```python
from build123d import *

# Parameters (mm, degrees)
SKETCH1_R             = 8
SKETCH1_R_2           = 4
BOSS_EXTRUDE1_DEPTH   = 9
BOSS_EXTRUDE1_2_DEPTH = 9
SKETCH2_R             = 4
BOSS_EXTRUDE3_DEPTH   = 9
FILLET1_R             = 1
SKETCH3_W             = 9
SKETCH3_H             = 9
SKETCH3_H_2           = 7
CUT_EXTRUDE1_DEPTH    = 214.789616212


with BuildPart() as part:
    # Sketch1 → Boss-Extrude1 (new body)
    with BuildSketch(Plane.XY):
        with Locations((-125, 0)):
            Circle(SKETCH1_R)
        with Locations((-125, 0)):
            Circle(SKETCH1_R_2, mode=Mode.SUBTRACT)
    extrude(amount=BOSS_EXTRUDE1_DEPTH)



with BuildPart() as body_2:
    # Sketch1 → Boss-Extrude1 2 (new body)
    with BuildSketch(Plane.XY):
        with Locations((125, 0)):
            Circle(SKETCH1_R)
        with Locations((125, 0)):
            Circle(SKETCH1_R_2, mode=Mode.SUBTRACT)
    extrude(amount=BOSS_EXTRUDE1_2_DEPTH)


with BuildPart() as part_1:
    add(part.part)

    add(body_2.part)  # Boss-Extrude3 merges body 2
    # Sketch2 → Boss-Extrude3 (add)
    with BuildSketch(Plane.XY):
        with BuildLine():
            Line((-175, -75), (125, -75))
            ThreePointArc((125, -75), (130.131670325, -43.377223009), (145.000000492, -14.999999344))
            ThreePointArc((145.000000492, -14.999999344), (143.981414944, 16.269784471), (113.235294528, 22.058823748))
            ThreePointArc((113.235294528, 22.058823748), (25.000000075, 0), (-63.235294395, 22.058823677))
            ThreePointArc((-63.235294395, 22.058823677), (-75.420498385, 24.996463372), (-87.499999896, 21.650635154))
            ThreePointArc((-87.499999896, 21.650635154), (-99.999999954, 18.301270189), (-112.500000024, 21.650635108))
            ThreePointArc((-112.500000024, 21.650635108), (-124.99999995, 25), (-137.49999989, 21.650635158))
            ThreePointArc((-137.49999989, 21.650635158), (-149.999999954, 18.301270189), (-162.50000003, 21.650635112))
            ThreePointArc((-162.50000003, 21.650635112), (-193.705072901, 16.586749162), (-195.000000551, -14.999999265))
            ThreePointArc((-195.000000551, -14.999999265), (-180.13167034, -43.377222962), (-175, -75))
        make_face()
        with Locations((125, 0)):
            Circle(SKETCH2_R, mode=Mode.SUBTRACT)
        with Locations((-175, 0)):
            Circle(SKETCH2_R, mode=Mode.SUBTRACT)
        with Locations((-125, 0)):
            Circle(SKETCH2_R, mode=Mode.SUBTRACT)
        with Locations((-75, 0)):
            Circle(SKETCH2_R, mode=Mode.SUBTRACT)
    extrude(amount=BOSS_EXTRUDE3_DEPTH)

    # Fillet1
    fillet1_edges = [part_1.edges().sort_by_distance(p)[0] for p in [
        (-175, -75, 4.5),
        (125, -75, 4.5),
    ]]
    fillet(fillet1_edges, radius=FILLET1_R)

    # Sketch3 → Cut-Extrude1 (cut, through all)
    with BuildSketch(Plane.XY):
        with Locations((-160.208548161, -70.5)):
            Rectangle(SKETCH3_W, SKETCH3_H)
        with Locations((-25.351798772, -70.5)):
            Rectangle(SKETCH3_W, SKETCH3_H)
        with Locations((109.504950616, -70.5)):
            Rectangle(SKETCH3_W, SKETCH3_H)
        with Locations((-160.208548161, -53.5)):
            Rectangle(SKETCH3_W, SKETCH3_H_2)
        with Locations((-25.351798772, -53.5)):
            Rectangle(SKETCH3_W, SKETCH3_H_2)
        with Locations((109.504950616, -53.5)):
            Rectangle(SKETCH3_W, SKETCH3_H_2)
    extrude(amount=CUT_EXTRUDE1_DEPTH, mode=Mode.SUBTRACT)


solid = part_1.part
```
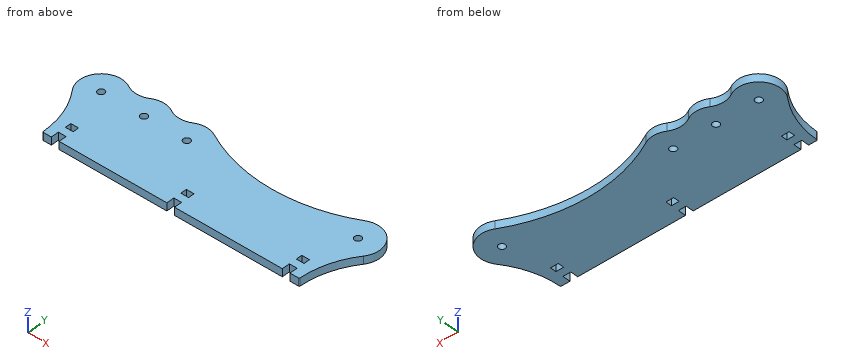
Check sheet for the modelled part. Datum: model origin and axes. Units: mm. Round coordinates to 2 decimals unless told otherwise and drop trailing zeros. Loops run counter-clockwise (first coordinate to the right, second up) from the corner with the lowest first, then second, coordinate; pieces in that order, holes last. Notation, with made-up numbers: (-23.75, 36.5) - (34.25, 36.5) arc R20 cw to (34.25, 62.5) - close; hole circle Ø10 at (-14.5, 59.5). An arc over 180 degrees is marked (long way). Answer as a JSON object with one key per item and string values. Group by question number.
Q1. Gauge pin test, flat ends, axial feed: P1, Ø4.5, axis at x = -23.5, z = 6.5, coming from the -Y side; P2, Ø2.5, axis at y = -70, z = 4, coming from the +X side; P3, Ø9, axis at x = -75, y = 0, coming from the -Z side; P4, Ø2, axis at y = -52.5, z = 6.5, coming from the +X side. Record the tip position at first contact, or that the pin passes through.
Q2. Sectioned sample at D-D, the plane y = -19. Enter the section's corners in (x, z), plus the area to 3 significant figures.
Q3. Sectioned sample at B-B, the plane x = -75. Enter the section's corners in (y, z).
Q4. Sectioned sample at A-A, the plane y = 13. Enter the section's corners in (x, z), plus the area to 3 significant figures.
Q5. Sectioned sample at C-C, the plane z = 3. Count the separate pieces of the cut face and the enclosed holes in it, plus the area to 3 significant figures.
Q6. Scan lines: line 1 along Y through (x, z) = (-125, 5); line 2 along X through (y, z) = (17.5, 6.75); line 3 along Y through (x, z) = (-151.5, 2). Record each from-to range of solid material in increasing order. Write a range as [from, to].
Solution:
{
 "1": {"P1": "stops at y = -66", "P2": "stops at x = 125.2", "P3": "stops at z = 0", "P4": "stops at x = 127.8"},
 "2": {"outline": "(-192.15, 0) - (142.15, 0) - (142.15, 9) - (-192.15, 9) - close", "area": "3,010 mm²"},
 "3": {"outline": "(-75, 0) - (-4, 0) - (-4, 9) - (-75, 9) - close; (4, 0) - (25, 0) - (25, 9) - (4, 9) - close"},
 "4": {"outline": "(-196.35, 0) - (-43.6, 0) - (-43.6, 9) - (-196.35, 9) - close; (93.6, 0) - (146.35, 0) - (146.35, 9) - (93.6, 9) - close", "area": "1,850 mm²"},
 "5": {"separate pieces": "1", "enclosed holes": "7", "area": "28,300 mm²"},
 "6": {"line 1": "y = [-75, -4], [4, 25]", "line 2": "x = [-192.85, -54.1], [104.1, 142.85]", "line 3": "y = [-75, 18.35]"}
}
